For this review, use the dimensioned drawing (mm, ordinates from the lowest corner) and the shaded views. A direction names the side the tool comes from. Give positions to 0.01 mm unless a question says otherwise; leave off trailing zeros. Order: outer loops, then holes, each group sorted by start corner. A loop starts at its lowest first (then second) coordinate and runs counter-clockwise, first axis right, second up. Notation, with made-up numbers: (68.5, 29.25) - (82.5, 29.25) arc R13 ccw to (82.5, 49.25) - close; hole circle Ø6 at (65.25, 63). An arc over 180 degrees is marked (long way). One line per item, written item: value.
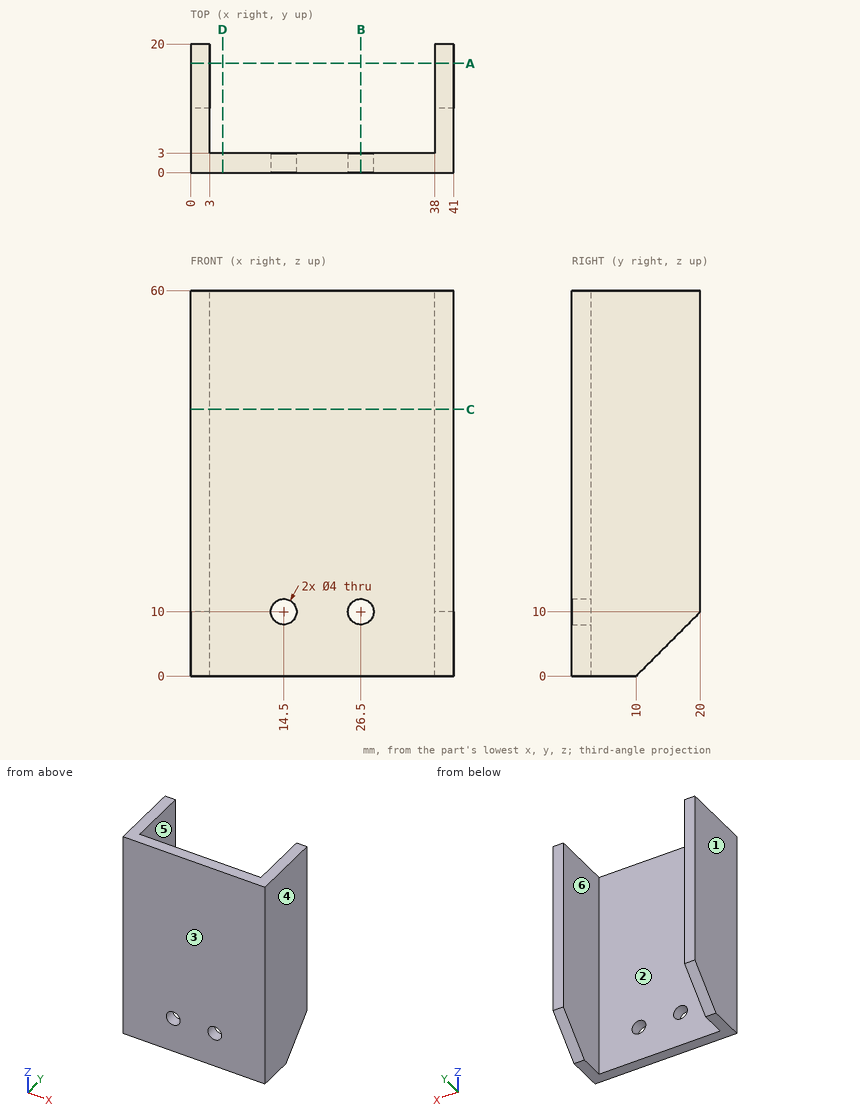
(1) For P1, Ø5, axis at x = 14.5, z = 10, coming from the +Y side, flat-tipped, find the tip position at first contact; note if it passes through.
Answers below:
P1: stops at y = 3
(2) Machinability: for the marked faces 1 and 2, which of the approach directions +Z, -Z, +X, -X, +Y, -Y give a long, thin tool a straight path to every point of the face, cutting with its end or side? Answer none if there is none.
Answers below:
face 1: +Z, -Z, -X, +Y, -Y
face 2: +Z, -Z, +Y
(3) Take a section at A-A (y = 17). Write out the cut boundary in (x, z).
Answers below:
outline: (0, 7) - (3, 7) - (3, 60) - (0, 60) - close; (38, 7) - (41, 7) - (41, 60) - (38, 60) - close
(4) Draft analysis for pull direction X (two halves, no side actions). For the marked faces 3, 4, 5 and 6, state which applies: pulls with the +X half, pulls with the -X half, needs draft (parallel to the pull), parting line crosses it, or undercut.
Answers below:
face 3: needs draft
face 4: pulls with the +X half
face 5: undercut
face 6: undercut
(5) Take a section at B-B (x = 26.5). Write out the cut boundary in (y, z).
Answers below:
outline: (0, 0) - (3, 0) - (3, 8) - (0, 8) - close; (0, 12) - (3, 12) - (3, 60) - (0, 60) - close
(6) Take a section at C-C (z = 41.5). Write out the cut boundary in (x, y), then the cut area to 3 significant figures.
Answers below:
outline: (0, 0) - (41, 0) - (41, 20) - (38, 20) - (38, 3) - (3, 3) - (3, 20) - (0, 20) - close
area: 225 mm^2
(7) Take a section at D-D (x = 5). Write out the cut boundary in (y, z), then the cut area to 3 significant figures.
Answers below:
outline: (0, 0) - (3, 0) - (3, 60) - (0, 60) - close
area: 180 mm^2
(8) Wall thickness on line 1 (X direction, y = 14, z = 57); line 2 (Z direction, x = 14.5, y = 1.15); line 3 (Y direction, x = 7, z = 34.5): over which ranges is each line inside the solid? List them lowest first. Write a range as from..to.
Answers below:
line 1: x = 0..3, 38..41
line 2: z = 0..8, 12..60
line 3: y = 0..3
